```python
from build123d import *

# Parameters (mm, degrees)
REDONDEO1_R                  = 2
CROQUIS2_R                   = 5
SALIENTE_EXTRUIR1_DEPTH      = 5
REDONDEO2_R                  = 1
CROQUIS3_R                   = 1.5
SALIENTE_EXTRUIR2_DEPTH      = 60
CROQUIS4_W                   = 16.15
CROQUIS4_H                   = 16.15
CROQUIS4_RX                  = 6
CROQUIS4_RY                  = 5.9
CORTAR_EXTRUIR1_DEPTH        = 117.5
CROQUIS5_W                   = 6
CROQUIS5_H                   = 28
SALIENTE_EXTRUIR3_DEPTH      = 6.5
CROQUIS6_W                   = 12
CROQUIS6_H                   = 4
CROQUIS6_W_2                 = 4
CROQUIS6_H_2                 = 11.8
CORTAR_EXTRUIR_L_MINA1_DEPTH = 8
CROQUIS7_R                   = 4.5
CORTAR_EXTRUIR2_DEPTH        = 8


with BuildPart() as part:
    # Croquis1 → Revolución1 (revolve)
    with BuildSketch(Plane.XY, mode=Mode.PRIVATE) as revoluci_n1_sk:
        Polygon((0, 0), (6.25, 0), (6.25, 117.5), (8.075, 117.5), (8.075, 157.5), (0, 157.5), align=None)
    revolve(revoluci_n1_sk.sketch.rotate(Axis((0, 0, 0), (0, -1, 0)), 90), axis=Axis((0, 0, 0), (0, -1, 0)))

    # Redondeo1
    # the kernel refuses this fillet: 2 mm, written as the material it takes off along each edge
    with BuildSketch(Plane(origin=(0, 117.5, 0), x_dir=(0, 0, 1), z_dir=(1, 0, 0))) as redondeo1_piece_1:
        with BuildLine():
            CenterArc((6.075, -1.992329039), REDONDEO1_R, 0, 84.980199868)
            Line((8.075, -1.992329039), (8.115, -1.992329039))
            Line((8.115, -1.992329039), (8.115, 0))
            Line((8.115, 0), (8.075, 0.04))
            ThreePointArc((8.075, 0.04), (7.1625, 0.04), (6.2535, 0.039846581))
            Line((6.2535, 0.039846581), (6.25, 0))
        make_face()
    revolve(axis=Axis((0, 117.5, 0), (0, -1, 0)), mode=Mode.SUBTRACT)

    # Croquis2 → Saliente-Extruir1 (add)
    with BuildSketch(Plane(origin=(0, 157.5, 0), x_dir=(1, 0, 0), z_dir=(0, 1, 0))):
        with Locations(Location((0, 0, 0), (0, 0, 270))):
            Circle(CROQUIS2_R)
    extrude(amount=SALIENTE_EXTRUIR1_DEPTH)

    # Redondeo2
    redondeo2_edges = [part.edges().sort_by_distance(p)[0] for p in [
        (0, 157.5, -8.075),
    ]]
    fillet(redondeo2_edges, radius=REDONDEO2_R)

    # Croquis3 → Saliente-Extruir2 (add)
    with BuildSketch(Plane(origin=(0, 162.5, 0), x_dir=(1, 0, 0), z_dir=(0, 1, 0))):
        with Locations(Location((0, 0, 0), (0, 0, 90))):
            Circle(CROQUIS3_R)
    extrude(amount=SALIENTE_EXTRUIR2_DEPTH)

    # Croquis4 → Cortar-Extruir1 (cut)
    with BuildSketch(Plane.XZ):
        Rectangle(CROQUIS4_W, CROQUIS4_H)
        with Locations(Location((0, 0), (0, 0, 180))):
            Ellipse(CROQUIS4_RX, CROQUIS4_RY, mode=Mode.SUBTRACT)
    extrude(amount=-CORTAR_EXTRUIR1_DEPTH, mode=Mode.SUBTRACT)

    # Croquis5 → Saliente-Extruir3 (add)
    with BuildSketch(Plane(origin=(0, 0, 0), x_dir=(0, 0, -1), z_dir=(1, 0, 0))):
        with Locations((0, 92)):
            Rectangle(CROQUIS5_W, CROQUIS5_H)
    extrude(amount=-SALIENTE_EXTRUIR3_DEPTH)

    # Croquis6 → Cortar-Extruir-Lámina1 (cut)
    with BuildSketch(Plane.XZ):
        Rectangle(CROQUIS6_W, CROQUIS6_H)
        Rectangle(CROQUIS6_W_2, CROQUIS6_H_2)
    extrude(amount=-CORTAR_EXTRUIR_L_MINA1_DEPTH, mode=Mode.SUBTRACT)

    # Croquis7 → Cortar-Extruir2 (cut)
    with BuildSketch(Plane.XZ):
        Circle(CROQUIS7_R)
    extrude(amount=-CORTAR_EXTRUIR2_DEPTH, mode=Mode.SUBTRACT)


solid = part.part
```
For this review, take the finished solid that the model builds, in its own axes (mm). A direction names the side the tool comes from. Round coordinates to 2 decimals unless told otherwise and drop trailing zeros. Order: outer loops, then holes, each group sorted by start corner. A loop starts at its lowest first (then second) coordinate and runs counter-clockwise, first axis right, second up.
Q1. Machinability: for faces 1 (the flat face through (-4, 0, 4)), 2 (the flat face through (-5, 157.5, -2)), which of the approach directions +Z, -Z, +X, -X, +Y, -Y give a long, thin tool a straight path to every point of the face, cutting with its end or side? Answer none if there is none.
Findings below:
face 1: +Z, -Z, +X, -X, -Y
face 2: +Y
Q2. Mouldability with a two-part tool opening along X and no side actions: class faces 3 (the cylindrical face through (-4.88, 159.96, -1.08)), 4 (the flat face through (0, 8, 0)), 5 (the flat face through (-6.5, 92, 0)), 6 (the flat face through (4, 0, -4)) as pulls with the +X half, pulls with the -X half, needs draft (parallel to the pull), parting line crosses it, or undercut.
Findings below:
face 3: parting line crosses it
face 4: undercut
face 5: pulls with the -X half
face 6: needs draft
Q3. Wall thickness on line 1 (Y direction, x = 0.5, z = -6.5); line 2 (Z direction, x = -0.25, y = 26.5); line 3 (Z direction, x = 7, y = 156.5): over which ranges is each line inside the solid? List them lowest first.
Findings below:
line 1: y = 117.54 to 157.5
line 2: z = -5.89 to 5.89
line 3: z = -4.03 to 4.03
Q4. Insertion check: P1, Ø1.7, axis at y = 4.5, z = 4.5, coming from the +X side; P2, Ø4, axis at y = 73, z = -3, coming from the -X side; P3, Ø3, axis at x = -1, y = 155, coming from the -Z side (3 decimals); P4, Ø6, axis at x = 4, y = 196, coming from the +Z side. Each pin has a flat end and moves straight along its axis. Give the tip position at first contact, or say it passes through.
Findings below:
P1: stops at x = 4.71
P2: stops at x = -5.91
P3: stops at z = -8.075
P4: stops at z = 1.12
Q5. We need section A-A, the plane y = 123. Give the boundary of the cut face in (x, z) (3 decimals), plus the area to 3 significant figures.
Findings below:
outline: circle Ø16.15 at (0, 0)
area: 205 mm2
